```python
from build123d import *

# Parameters (mm, degrees)
SKETCH1_R           = 3.3
BOSS_EXTRUDE1_DEPTH = 4.7625


with BuildPart() as part:
    # Sketch1 → Boss-Extrude1 (new body)
    with BuildSketch(Plane.XY):
        with BuildLine():
            Line((-508.291723206, -95.594257619), (-487.660025711, -89.447897876))
            Line((-487.660025711, -89.447897876), (-496.962426186, -77.649232083))
            Line((-496.962426186, -77.649232083), (-512.277542982, -82.204928563))
            ThreePointArc((-512.277542982, -82.204928563), (-516.980664668, -90.89290993), (-508.291723206, -95.594257619))
        make_face()
        with Locations(Location((-510.286, -88.9, 0), (0, 0, 180))):
            Circle(SKETCH1_R, mode=Mode.SUBTRACT)
    extrude(amount=BOSS_EXTRUDE1_DEPTH)


solid = part.part
```
Geometry check sheet. Reference: the model listing, model coordinates, mm. Give positions to 0.01 mm unless a question says otherwise; leave off trailing zeros. Write each loop counter-clockwise with the first axis right and the second up, starting at its lowest first coordinate (ties: lowest second). Pieces come first, ordered by that corner, then holes.
1) Material ranges on L1, parallel to X at y = -87.5, z = 4; L2, parallel to X at y = -88.9, z = 3.6; L3, parallel to Y at x = -509.25, z = 0.3, recorded low to high.
2) Section check D-D, the plane x = -501.5. Record the boundary of the cut face in (y, z).
3) Section check A-A, the plane y = -87. Record the boundary of the cut face in (x, z).
4) Section check C-C, the plane y = -88.9. Record the boundary of the cut face in (x, z).
5) Release check for a two-part mould opening along X. For faces 1 (the cylindrical face through (-512.06, -91.683, 2.348)), 2 (the flat face through (-503, -87, 4.762)), 3 (the flat face through (-492.246, -83.631, 2.348)) record: pulls with the +X half, pulls with the -X half, needs draft (parallel to the pull), parting line crosses it, or undercut.
6) Section check B-B, the plane z = 3.9. Record the boundary of the cut face in (x, y) (3 decimals), and give its area (3 significant figures).
Computed:
1. L1: x = -517.13 to -513.27, -507.3 to -489.2
1. L2: x = -517.27 to -513.59, -506.99 to -488.09
1. L3: y = -95.81 to -92.03, -85.77 to -81.3
2. outline: (-93.57, 0) - (-79, 0) - (-79, 4.76) - (-93.57, 4.76) - close
3. outline: (-517.01, 0) - (-512.98, 0) - (-512.98, 4.76) - (-517.01, 4.76) - close; (-507.59, 0) - (-489.59, 0) - (-489.59, 4.76) - (-507.59, 4.76) - close
4. outline: (-517.27, 0) - (-513.59, 0) - (-513.59, 4.76) - (-517.27, 4.76) - close; (-506.99, 0) - (-488.09, 0) - (-488.09, 4.76) - (-506.99, 4.76) - close
5. face 1: undercut
5. face 2: needs draft
5. face 3: pulls with the +X half
6. outline: (-512.278, -82.205) arc R6.985 ccw to (-508.292, -95.594) - (-487.66, -89.448) - (-496.962, -77.649) - close; hole circle Ø6.6 at (-510.286, -88.9)
6. area: 304 mm2
